from build123d import *

# Parameters (mm, degrees)
SKETCH2_R           = 2.125
BOSS_EXTRUDE1_DEPTH = 9
SKETCH2_3_W         = 143.4775
SKETCH2_3_H         = 11.945
SKETCH2_3_R         = 1.5
BOSS_EXTRUDE2_DEPTH = 5.975
BOSS_EXTRUDE3_DEPTH = 6
SKETCH7_R           = 4.45
CUT_EXTRUDE4_DEPTH  = 138
CUT_EXTRUDE6_DEPTH  = 5
CUT_EXTRUDE7_DEPTH  = 5


with BuildPart() as part:
    # Sketch2 → Boss-Extrude1 (new, symmetric)
    with BuildSketch(Plane.XY):
        with BuildLine():
            Line((145.4775, 14.0125), (145.4775, 11.945))
            Line((145.4775, 11.945), (145.4775, 0))
            Line((145.4775, 0), (145.4775, -2.0675))
            ThreePointArc((145.4775, -2.0675), (145.623946609, -2.421053391), (145.9775, -2.5675))
            Line((145.9775, -2.5675), (198.1775, -2.5675))
            ThreePointArc((198.1775, -2.5675), (198.531053391, -2.421053391), (198.6775, -2.0675))
            Line((198.6775, -2.0675), (198.6775, 0))
            Line((198.6775, 0), (204.343857791, 0))
            ThreePointArc((204.343857791, 0), (206.701098803, 0.976401197), (207.6775, 3.333642209))
            Line((207.6775, 3.333642209), (207.6775, 6.708857791))
            ThreePointArc((207.6775, 6.708857791), (206.701098803, 9.066098803), (204.343857791, 10.0425))
            Line((204.343857791, 10.0425), (200.377364582, 10.0425))
            ThreePointArc((200.377364582, 10.0425), (200.021766481, 10.074366369), (199.6775, 10.168950009))
            Line((199.6775, 10.168950009), (198.6775, 10.5425))
            Line((198.6775, 10.5425), (198.6775, 16.9325))
            ThreePointArc((198.6775, 16.9325), (198.531053391, 17.286053391), (198.1775, 17.4325))
            Line((198.1775, 17.4325), (154.8775, 17.4325))
            ThreePointArc((154.8775, 17.4325), (154.523946609, 17.286053391), (154.3775, 16.9325))
            Line((154.3775, 16.9325), (154.3775, 15.0125))
            ThreePointArc((154.3775, 15.0125), (154.231053391, 14.658946609), (153.8775, 14.5125))
            Line((153.8775, 14.5125), (145.9775, 14.5125))
            ThreePointArc((145.9775, 14.5125), (145.623946609, 14.366053391), (145.4775, 14.0125))
        make_face()
        with Locations((203.0525, 5.02125)):
            Circle(SKETCH2_R, mode=Mode.SUBTRACT)
    extrude(amount=BOSS_EXTRUDE1_DEPTH, both=True)

    # Sketch2<3> → Boss-Extrude2 (add, symmetric)
    with BuildSketch(Plane.XY):
        with Locations((73.73875, 5.9725)):
            Rectangle(SKETCH2_3_W, SKETCH2_3_H)
        with Locations((5.5, 5.9725)):
            Circle(SKETCH2_3_R, mode=Mode.SUBTRACT)
    extrude(amount=BOSS_EXTRUDE2_DEPTH, both=True)

    # Sketch2<4> → Boss-Extrude3 (add, symmetric)
    with BuildSketch(Plane.XY):
        with BuildLine():
            Line((2, 0), (2, 11.945))
            Line((2, 11.945), (1, 11.945))
            ThreePointArc((1, 11.945), (0.292893219, 11.652106781), (0, 10.945))
            Line((0, 10.945), (0, 1))
            ThreePointArc((0, 1), (0.292893219, 0.292893219), (1, 0))
            Line((1, 0), (2, 0))
        make_face()
    extrude(amount=BOSS_EXTRUDE3_DEPTH, both=True)

    # Sketch7 → Cut-Extrude4 (cut)
    with BuildSketch(Plane.ZY):
        with Locations((0, 5.9725)):
            Circle(SKETCH7_R)
    extrude(amount=-CUT_EXTRUDE4_DEPTH, mode=Mode.SUBTRACT)

    # Sketch8 → Cut-Extrude6 (cut, symmetric)
    with BuildSketch(Plane.XY.offset(9)):
        Polygon((198.6775, 10.5425), (211.452070609, 15.905902501), (207.012502563, -2.059702975), (198.6775, 0), align=None)
    extrude(amount=CUT_EXTRUDE6_DEPTH, both=True, mode=Mode.SUBTRACT)

    # Sketch10 → Cut-Extrude7 (cut, symmetric)
    with BuildSketch(Plane(origin=(0, 0, -9), x_dir=(-1, 0, 0), z_dir=(0, 0, -1))):
        Polygon((-198.6775, 10.5425), (-218.686725566, 39.11278538), (-201.443333916, -35.592944689), (-198.6775, 0), align=None)
    extrude(amount=CUT_EXTRUDE7_DEPTH, both=True, mode=Mode.SUBTRACT)


solid = part.part
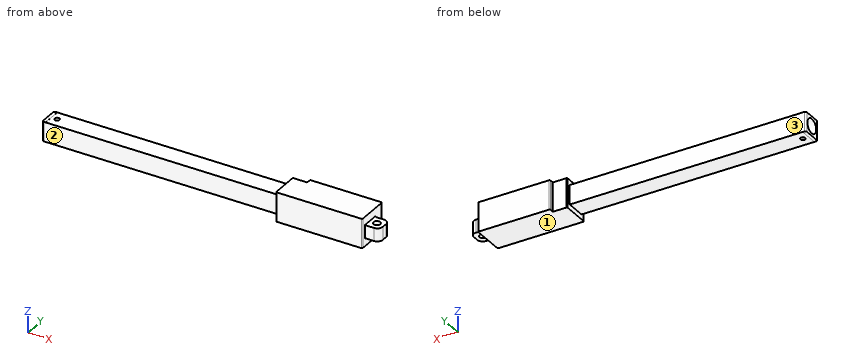
Could you check a few things on this model? Use its own coordinates, in mm. Face numbers are marked on the shaded views. A direction names the side the tool comes from. Coordinates: 2 decimals unless noted, no trailing zeros.
1. For the marked faces 1, 2 and 3, which set-ups out of +Z, -Z, +X, -X, +Y, -Y let a thin tool reach every point of the face, with its end or its side?
2. For P1, Ø2.5, axis at x = 202.5, y = 4.5, coming from the +Z side; P2, Ø8, axis at x = 31, z = 6.5, coming from the -Y side; P3, Ø4, axis at y = 11, z = 3, coming from the +X side; P4, Ø1.5, axis at x = 105.5, y = 2.5, coming from the +Z side (3 decimals), each with a flat end and sliding along its axis, tell me the tip position at first contact or that it passes through.
3. I need wall thicknesses on L1, parallel to Y at x = 5.5, z = 5.2 (1 decimal); L2, parallel to Y at x = 109.5, z = 0 (1 decimal); L3, parallel to X at y = -1.5, z = 6. Which ranges of each line are inside material? Lowest first, please.
Computed values:
1. face 1: -Z, +X, -X, +Y, -Y
1. face 2: +Z, -Z, -X, -Y
1. face 3: +Z, -Z, -X, +Y
2. P1: passes through
2. P2: stops at y = 0
2. P3: stops at x = 206.77
2. P4: stops at z = 5.975
3. L1: y = 0 to 4.5, 7.5 to 11.9
3. L2: y = 0 to 1.5, 10.4 to 11.9
3. L3: x = 145.48 to 198.68
